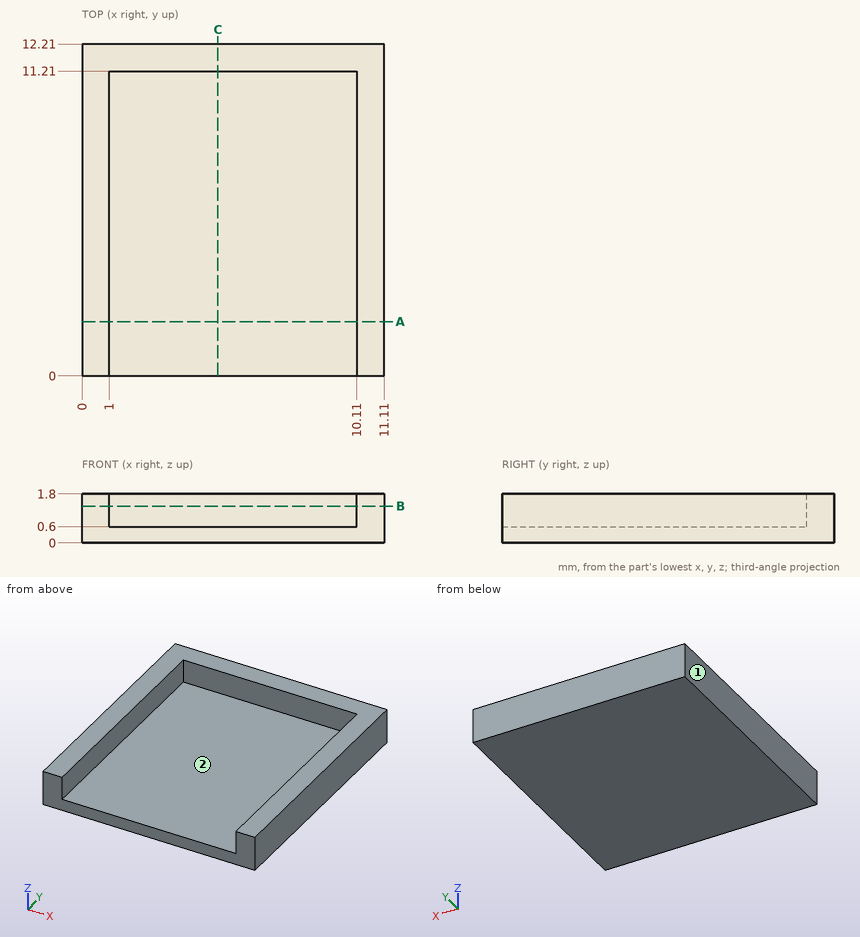
Print and shaded views of the part. All mm, measured from the part's lowest x, y and z. A direction names the side the tool comes from. Coordinates: 2 decimals unless noted, no trailing zeros. Order: outer loops, then holes, each group sorted by start corner. A loop starts at its lowest first (then second) coordinate and runs counter-clockwise, first axis right, second up. Notation, with made-up numbers: (21.25, 84) -> (55.25, 84) arc R12 cw to (55.25, 98) -> close; hole circle Ø11 at (27.25, -35). An arc over 180 degrees is marked (long way). Use one line per item in the form item = value. Start each with the question number.
1) Band-saw the part on B-B on z = 1.35. Give the cut face in (x, y).
2) Band-saw the part on C-C on x = 5. Give the cut face in (y, z), then the cut area to 3 significant figures.
3) Drill centre lines: L1, parallel to X at y = 11, z = 1.4; L2, parallel to Y at x = 2, z = 1.1; L3, parallel to Z at x = 5.25, y = 7.25. Where is each one in solid material? Low to high. Write a range as [from, to].
4) Tool access for the marked faces 1 and 2: list every direction of +Z, -Z, +X, -X, +Y, -Y with a clear straight run to the whole face (end or side of a thin tool).
5) Band-saw the part on A-A on y = 2. Give the cut face in (x, z).
6) Drop a flat-ended pin along its axis: pin 1 (2.5 mm diameter, centred on x = 5.5, y = 4.5, fed in from +Z). Give the stop position or say it passes through.
Entries:
q1.outline = (0, 0) -> (1, 0) -> (1, 11.21) -> (10.11, 11.21) -> (10.11, 0) -> (11.11, 0) -> (11.11, 12.21) -> (0, 12.21) -> close
q2.outline = (0, 0) -> (12.21, 0) -> (12.21, 1.8) -> (11.21, 1.8) -> (11.21, 0.6) -> (0, 0.6) -> close
q2.area = 8.53 mm2
q3.L1 = [0, 1], [10.11, 11.11]
q3.L2 = [11.21, 12.21]
q3.L3 = [0, 0.6]
q4.face_1 = +Z, -Z, -X, +Y, -Y
q4.face_2 = +Z, -Y
q5.outline = (0, 0) -> (11.11, 0) -> (11.11, 1.8) -> (10.11, 1.8) -> (10.11, 0.6) -> (1, 0.6) -> (1, 1.8) -> (0, 1.8) -> close
q6.pin_1 = 0.6
